Geometry: final body of the model. Coordinates: model frame, mm. A direction names the side the tool comes from. Give positions to 0.01 mm unless a question says otherwise; leave off trailing zeros. Order: outer loops, then holes, each group sorted by start corner. A loop starts at its lowest first (then second) coordinate and runs counter-clockwise, first axis right, second up. Notation, with made-up numbers: (15.25, -30) -> (50.25, -30) arc R18 cw to (50.25, -19) -> close; hole circle Ø8 at (63, -17). An arc over 180 degrees is marked (long way). Answer in a Markdown table with one row per item. Add a question column.
Q1. Cut plane A-A on y = 4.5. Return the cut outline in (x, z).
Q2. Set-up query: faces 4 (the face through (0, 0, 0)), 5 (the face through (-0.759, 8.107, -5.473)). Return all of +Z, -Z, +X, -X, +Y, -Y with unobstructed straight access to the full face (end or side cutting, diameter ignored); none if empty.
Q3. Cut plane D-D on x = 2.5. Return the cut outline in (y, z), and give its area (3 significant figures).
Q4. Cut plane B-B on z = -8.89. Return the cut outline in (x, y).
Q5. Contact query for flat-ended pins moving along their axis: P1, Ø5.5, axis at x = 0.5, z = 8, coming from the +Y side; P2, Ø3, axis at x = 2.5, z = 2, coming from the +Y side; P3, Ø1.5, axis at x = 2.5, z = 9.5, coming from the +Y side. Output: stop coordinate, or through.
Q6. Line query: line 1 along Z through (x, y) = (0, 8.05); line 2 along X through (y, z) = (8.2, -8.89); line 3 along Y through (x, z) = (4.5, -12.5). Output: solid intervals per line, ascending. Write a range as from..to.
Q7. Cut plane C-C on x = 0. Return the cut outline in (y, z).
Q8. Pull-direction query (X, two-part tool) for faces 1 (the face through (-6, 1, 0)), 2 (the face through (0, 7.6, 9)), 3 (the face through (0, 1.6, 0)); classes: +X half, -X half, draft (parallel to the pull), parting line (faces both ways), or undercut.
Autodesk Inventor part; units mm, degrees
ref_plane "YZ Plane" through (0, 0, 0) normal (1, 0, 0) x (0, 1, 0)
ref_plane "XZ Plane" through (0, 0, 0) normal (0, 1, 0) x (-1, 0, 0)
ref_plane "XY Plane" through (0, 0, 0) normal (0, 0, 1) x (1, 0, 0)
sketch "Sketch1" plane through (0, 0, 0) normal (0, 1, 0) x (-1, 0, 0)
  line L0 (-6, -15) -> (-6, 15)
  line L1 (-6, 15) -> (6, 15)
  line L2 (6, 15) -> (6, -15)
  line L3 (6, -15) -> (-6, -15)
  line L4 (-6, -15) -> (6, 15) construction
  line L5 (-6, 15) -> (6, -15) construction
  line L6 (-6, -15) -> (24, -15) construction
  point P0 (0, 0)
  dimension "d0" = 30
  dimension "d1" = 90
  dimension "d2" = 12
extrude "Extrusion1" add sketch "Sketch1" along normal blind 1.6
sketch "Sketch2" plane through (0, 1.6, 0) normal (0, 1, 0) x (1, 0, 0)
  line L0 (0, 0) -> (0, -8.89)
  line L1 (0, 0) -> (8.89, 0) construction
  line L2 (0, -8.89) -> (0, 8.89)
  circle A0 centre (0, -8.89) radius 4.75
  circle A1 centre (0, 8.89) radius 4.75
  dimension "d5" = 8.89
  dimension "d6" = 90
  dimension "d7" = 17.78
  dimension "d8" = 0
  dimension "d9" = 9.5
  dimension "d10" = 9.5
extrude "Extrusion2" add sketch "Sketch2" along normal blind 7
sketch "Sketch3" plane through (0, 8.6, 8.89) normal (0, 1, 0) x (1, 0, 0)
  circle A0 centre (0, 0) radius 3.5
  line L0 (0, 8.89) -> (0, 17.78)
  circle A1 centre (0, 17.78) radius 3.5
  dimension "d13" = 7
  dimension "d14" = 8.89
  dimension "d15" = 7
extrude "Extrusion3" cut sketch "Sketch3" against normal blind 1
properties part number "Sonar"
Completed:
| question | item | result |
|---|---|---|
| 1 | outline | circle Ø9.5 at (0, -8.89); circle Ø9.5 at (0, 8.89) |
| 2 | face 4 | +Z, -Z, +X, -X, -Y |
| 2 | face 5 | +Y |
| 3 | outline | (0, -15) -> (1.6, -15) -> (1.6, -12.93) -> (8.6, -12.93) -> (8.6, -11.34) -> (7.6, -11.34) -> (7.6, -6.44) -> (8.6, -6.44) -> (8.6, -4.85) -> (1.6, -4.85) -> (1.6, 4.85) -> (8.6, 4.85) -> (8.6, 6.44) -> (7.6, 6.44) -> (7.6, 11.34) -> (8.6, 11.34) -> (8.6, 12.93) -> (1.6, 12.93) -> (1.6, 15) -> (0, 15) -> close |
| 3 | area | 151 mm² |
| 4 | outline | (-6, 0) -> (6, 0) -> (6, 1.6) -> (4.75, 1.6) -> (4.75, 8.6) -> (3.5, 8.6) -> (3.5, 7.6) -> (-3.5, 7.6) -> (-3.5, 8.6) -> (-4.75, 8.6) -> (-4.75, 1.6) -> (-6, 1.6) -> close |
| 5 | P1 | stops at y = 8.6 |
| 5 | P2 | stops at y = 1.6 |
| 5 | P3 | stops at y = 7.6 |
| 6 | line 1 | z = -13.64..-12.39, -5.39..-4.14, 4.14..5.39, 12.39..13.64 |
| 6 | line 2 | x = -4.75..-3.5, 3.5..4.75 |
| 6 | line 3 | y = 0..1.6 |
| 7 | outline | (0, -15) -> (1.6, -15) -> (1.6, -13.64) -> (8.6, -13.64) -> (8.6, -12.39) -> (7.6, -12.39) -> (7.6, -5.39) -> (8.6, -5.39) -> (8.6, -4.14) -> (1.6, -4.14) -> (1.6, 4.14) -> (8.6, 4.14) -> (8.6, 5.39) -> (7.6, 5.39) -> (7.6, 12.39) -> (8.6, 12.39) -> (8.6, 13.64) -> (1.6, 13.64) -> (1.6, 15) -> (0, 15) -> close |
| 8 | face 1 | -X half |
| 8 | face 2 | undercut |
| 8 | face 3 | draft |
